The model under review builds one solid part; all positions refer to its coordinate system, in mm. Coordinates: 2 decimals unless noted, no trailing zeros. Order: outer loops, then holes, each group sorted by start corner. A loop starts at its lowest first (then second) coordinate and runs counter-clockwise, first axis right, second up. Notation, with made-up numbers: (-24.5, 64.5) -> (24.5, 64.5) arc R19 ccw to (24.5, 74.5) -> close; hole circle Ø1 at (32.5, 59.5). An arc over 180 degrees is marked (long way). Use one line per item in the form item = value.
from build123d import *

# Parameters (mm, degrees)
F0_R          = 50.8
F1_DEPTH      = 50.8
F1_DEPTH_BACK = 50.8
F4_START      = -50.8
F2_R          = 50.8
F4_DEPTH      = 101.6
F5_START      = -50.8
F3_R          = 50.8
F5_DEPTH      = 101.6


with BuildPart() as f1:
    # F0 (on Top) → F1 (new body, two sides)
    with BuildSketch(Plane.XY) as f1_sk:
        Circle(F0_R)
    extrude(amount=F1_DEPTH)
    extrude(f1_sk.sketch, amount=-F1_DEPTH_BACK)

    # F2 (on Front) → F4 (intersect)
    with BuildSketch(Plane.XZ.offset(F4_START)):
        Circle(F2_R)
    extrude(amount=F4_DEPTH, mode=Mode.INTERSECT)

    # F3 (on Right) → F5 (intersect)
    with BuildSketch(Plane.YZ.offset(F5_START)):
        Circle(F3_R)
    extrude(amount=F5_DEPTH, mode=Mode.INTERSECT)


solid = f1.part
Item 1: To check wall thickness, follow L1, parallel to Z at x = -31.5, y = -13.5; L2, parallel to Z at x = 19.5, y = 13; L3, parallel to Y at x = -2, z = 29.5. State the ranges of each line that lie inside material, in increasing order. Write a range as from..to.
Results found:
L1 = -39.85..39.85
L2 = -46.91..46.91
L3 = -41.36..41.36
Item 2: We need section A-A (y = -3). Write out the cut boundary in (x, z), plus the area to 3 significant figures.
Results found:
outline = (-50.71, -3) arc R50.8 ccw to (-3, -50.71) -> (3, -50.71) arc R50.8 ccw to (50.71, -3) -> (50.71, 3) arc R50.8 ccw to (3, 50.71) -> (-3, 50.71) arc R50.8 ccw to (-50.71, 3) -> close
area = 8,110 mm²
Item 3: Draft analysis for pull direction X (two halves, no side actions). For faces 1 (the face through (35.524, 0.503, -36.314)), 2 (the face through (-36.314, -35.524, 0.503)), state which applies: released by +X, released by -X, zero draft, split by the parting line, or undercut.
Results found:
face_1 = released by +X
face_2 = released by -X
Item 4: Clearance check with flat-ended pins moving along their axes: pin 1 (5 mm diameter, centred on x = -33, y = 15, fed in from +Z) (3 decimals); pin 2 (2 mm diameter, centred on y = -3.5, z = 8.5, fed in from -X); pin 3 (5 mm diameter, centred on x = -21.5, z = 36.5, fed in from +Y). State where each tip first meets the part, or that it passes through.
Results found:
pin_1 = 40.625
pin_2 = -50.24
pin_3 = 37.74
Item 5: We need section B-B (z = -15). Write out the cut boundary in (x, y), plus the area to 3 significant figures.
Results found:
outline = (-48.53, -15) arc R50.8 ccw to (-15, -48.53) -> (15, -48.53) arc R50.8 ccw to (48.53, -15) -> (48.53, 15) arc R50.8 ccw to (15, 48.53) -> (-15, 48.53) arc R50.8 ccw to (-48.53, 15) -> close
area = 7,930 mm²
Item 6: We need section D-D (y = -43.5). Write out the cut boundary in (x, z), plus the area to 3 significant figures.
Results found:
outline = (-26.24, -26.24) -> (26.24, -26.24) -> (26.24, 26.24) -> (-26.24, 26.24) -> close
area = 2,750 mm²
Item 7: We need section C-C (x = 40.5). Write out the cut boundary in (y, z), plus the area to 3 significant figures.
Results found:
outline = (-30.67, -30.67) -> (30.67, -30.67) -> (30.67, 30.67) -> (-30.67, 30.67) -> close
area = 3,760 mm²
